Input: part model. Units: mm. Frame: model coordinates. A direction names the side the tool comes from. Coordinates: 2 decimals unless noted, no trailing zeros. Write each loop counter-clockwise with the first axis right and the second up, starting at its lowest first coordinate (ties: lowest second). Pieces come first, ordered by that corner, then holes. Notation, with made-up numbers: M 52,-7 L 78,-7 A13 ccw 78,11 Z; hole C 30.5,2 d7. An arc over 180 degrees is marked long. Use CSV: the item, a comma, the result in double quotes.
```python
from build123d import *

# Parameters (mm, degrees)
F0_W      = 330.2095
F0_H      = 512.4196
F1_DEPTH  = 25.4
F2_DEPTH  = 22.225
F3_W      = 101.6
F3_H      = 101.6
F4_DEPTH  = 12.7
F6_DEPTH  = 38.1
F7_W      = 228.6
F7_H      = 15.875
F8_DEPTH  = 127
F9_W      = 228.6
F9_H      = 15.875
F10_DEPTH = 127
F11_R     = 31.75


with BuildPart() as f1:
    # F0 (on Front) → F1 (new body)
    with BuildSketch(Plane.XZ):
        with BuildLine():
            Line((184.15475, -262.5598), (184.15475, 262.5598))
            ThreePointArc((184.15475, 262.5598), (180.435006, 271.540056), (171.45475, 275.2598))
            Line((171.45475, 275.2598), (-171.45475, 275.2598))
            ThreePointArc((-171.45475, 275.2598), (-180.435006, 271.540056), (-184.15475, 262.5598))
            Line((-184.15475, 262.5598), (-184.15475, -262.5598))
            ThreePointArc((-184.15475, -262.5598), (-180.435006, -271.540056), (-171.45475, -275.2598))
            Line((-171.45475, -275.2598), (171.45475, -275.2598))
            ThreePointArc((171.45475, -275.2598), (180.435006, -271.540056), (184.15475, -262.5598))
        make_face()
        Rectangle(F0_W, F0_H, mode=Mode.SUBTRACT)
    extrude(amount=F1_DEPTH)

    # F0 (on Front) → F2 (join)
    with BuildSketch(Plane.XZ):
        Rectangle(F0_W, F0_H)
    extrude(amount=F2_DEPTH)

    # F3 (on face) → F4 (join)
    with BuildSketch(Plane.XZ):
        Rectangle(F3_W, F3_H)
    extrude(amount=-F4_DEPTH)

    # F5 (on Right) → F6 (join, symmetric)
    with BuildSketch(Plane.YZ):
        Polygon((12.7, 31.75), (12.7, -31.75), (36.226559, -300.6598), (-76.2, -300.6598), (-76.2, -316.5348), (152.4, -316.5348), (152.4, -300.6598), (76.2, -300.6598), align=None)
    extrude(amount=F6_DEPTH, both=True)

    # F7 (on face) → F8 (join)
    with BuildSketch(Plane.YZ.offset(38.1)):
        with Locations((38.1, -308.5973)):
            Rectangle(F7_W, F7_H)
    extrude(amount=F8_DEPTH)

    # F9 (on face) → F10 (join)
    with BuildSketch(Plane(origin=(-38.1, 0, 0), x_dir=(0, -1, 0), z_dir=(-1, 0, 0))):
        with Locations((-38.1, -308.5973)):
            Rectangle(F9_W, F9_H)
    extrude(amount=F10_DEPTH)

    # F11
    f11_edges = [f1.edges().sort_by_distance(p)[0] for p in [
        (-165.1, 152.4, -308.5973),
        (165.1, 152.4, -308.5973),
        (165.1, -76.2, -308.5973),
        (-165.1, -76.2, -308.5973),
    ]]
    fillet(f11_edges, radius=F11_R)


solid = f1.part
```
1. Access query for faces 1 (the flat face through (-178, -25.4, 1)), 2 (the flat face through (-2, -22.225, 4)), 3 (the cylindrical face through (155.6, -67.1, -308.5)), 4 (the cylindrical face through (180.336, -12.522, -271.638)), 5 (the flat face through (-1, 6, 50.8)). Directions: +Z, -Z, +X, -X, +Y, -Y. A direction counts if a zero-diameter tool reaches every point of the face in a straight line with its end or side. Return the directions, or none.
Resolved:
face 1,"+Z, +X, -X, -Y"
face 2,"-Y"
face 3,"+Z, -Z, +X, -Y"
face 4,"-Z, +X, +Y, -Y"
face 5,"+Z, +X, -X, +Y"
2. Section C-C (z = -38). Return loops of the section in (x, y) (3 decimals), then the cut area to 3 significant figures.
Resolved:
outline,"M -184.155,-25.4 L -165.105,-25.4 L -165.105,-22.225 L 165.105,-22.225 L 165.105,-25.4 L 184.155,-25.4 L 184.155,0 L 50.8,0 L 50.8,12.7 L -50.8,12.7 L -50.8,0 L -184.155,0 Z; M -38.1,13.247 L 38.1,13.247 L 38.1,26.024 L -38.1,26.024 Z"
area,"10,600 mm^2"
3. Contact query for flat-ended pins moving along their axis: pin 1 Ø2 at (x, z) = (87, 58) entering from +Y; pin 2 Ø8 at (y, z) = (7.5, -312.5) entering from +X; pin 3 Ø12 at (x, z) = (-21.5, -10) entering from +Y. Output: stop coordinate, or through.
Resolved:
pin 1,"stops at y = 0"
pin 2,"stops at x = 165.1"
pin 3,"stops at y = 21.82"
4. Mould query, pull axis Y, two halves, no side actions, for faces 6 (the flat face through (-1, 12.7, 35)), 7 (the cylindrical face through (-155.6, 143.3, -308.5)), 8 (the flat face through (-2, -13, -275.26)). Classes: pulls with the +Y half, pulls with the -Y half, needs draft (parallel to the pull), parting line crosses it, or undercut.
Resolved:
face 6,"undercut"
face 7,"pulls with the +Y half"
face 8,"needs draft"
5. Material intervals for line 1 (X direction, y = 63, z = -234.5); line 2 (Y direction, x = -72, z = -58) (3 decimals); line 3 (Z direction, x = 65, y = 26), sorted ascending. Write a range as [from, to].
Resolved:
line 1,"x = [-38.1, 38.1]"
line 2,"y = [-22.225, 0]"
line 3,"z = [-316.53, -300.66]"
6. Section D-D (x = -7.5). Return loops of the section in (y, z) (3 decimals), then the cut area to 3 significant figures.
Resolved:
outline,"M -76.2,-316.535 L 152.4,-316.535 L 152.4,-300.66 L 76.2,-300.66 L 12.7,31.75 L 12.7,50.8 L 0,50.8 L 0,275.26 L -25.4,275.26 L -25.4,256.21 L -22.225,256.21 L -22.225,-256.21 L -25.4,-256.21 L -25.4,-275.26 L 0,-275.26 L 0,-50.8 L 12.7,-50.8 L 12.7,-31.75 L 36.227,-300.66 L -76.2,-300.66 Z"
area,"24,700 mm^2"
7. Section B-B (x = 121.5). Return loops of the section in (y, z) (3 decimals), then the cut area to 3 significant figures.
Resolved:
outline,"M -76.2,-316.535 L 152.4,-316.535 L 152.4,-300.66 L -76.2,-300.66 Z; M -25.4,-275.26 L 0,-275.26 L 0,275.26 L -25.4,275.26 L -25.4,256.21 L -22.225,256.21 L -22.225,-256.21 L -25.4,-256.21 Z"
area,"16,000 mm^2"
8. Section A-A (y = -16). Return loops of the section in (x, z).
Resolved:
outline,"M -184.15,-262.56 A12.7 ccw -171.45,-275.26 L 171.45,-275.26 A12.7 ccw 184.15,-262.56 L 184.15,262.56 A12.7 ccw 171.45,275.26 L -171.45,275.26 A12.7 ccw -184.15,262.56 Z; M -165.1,-316.53 L 165.1,-316.53 L 165.1,-300.66 L -165.1,-300.66 Z"
